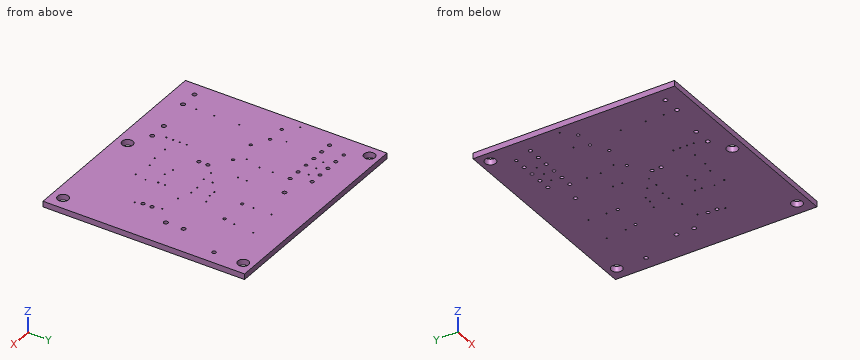
Autodesk Inventor part; units mm, degrees
ref_plane "YZ Plane" through (0, 0, 0) normal (1, 0, 0) x (0, 1, 0)
ref_plane "XZ Plane" through (0, 0, 0) normal (0, 1, 0) x (-1, 0, 0)
ref_plane "XY Plane" through (0, 0, 0) normal (0, 0, 1) x (1, 0, 0)
sketch "Sketch1" plane through (0, 0, 0) normal (0, 0, 1) x (1, 0, 0)
  line L0 (0, 0) -> (61.575, 0)
  line L1 (61.575, 0) -> (61.575, 56.82)
  line L2 (61.575, 56.82) -> (0, 56.82)
  line L3 (0, 56.82) -> (0, 0)
  circle A0 centre (10.16, 30.48) radius 0.405
  circle A1 centre (5.08, 30.48) radius 0.405
  circle A2 centre (22.23, 27.94) radius 0.405
  circle A3 centre (14.61, 27.94) radius 0.405
  circle A4 centre (44.45, 40.01) radius 0.405
  circle A5 centre (36.83, 40.01) radius 0.405
  circle A6 centre (27.3, 24.13) radius 0.51
  circle A7 centre (27.3, 21.59) radius 0.51
  circle A8 centre (49.53, 22.86) radius 0.51
  circle A9 centre (49.53, 20.32) radius 0.51
  circle A10 centre (27.3, 45.72) radius 0.55
  circle A11 centre (57.79, 45.72) radius 0.55
  circle A12 centre (4.57, 43.61) radius 0.5
  circle A13 centre (6.27, 48.69) radius 0.43
  circle A14 centre (7.98, 43.61) radius 0.5
  circle A15 centre (9.68, 48.69) radius 0.5
  circle A16 centre (11.38, 43.61) radius 0.5
  circle A17 centre (13.08, 48.69) radius 0.5
  circle A18 centre (14.78, 43.61) radius 0.43
  circle A19 centre (16.48, 48.69) radius 0.5
  circle A20 centre (18.19, 43.61) radius 0.5
  circle A21 centre (19.89, 48.69) radius 0.5
  circle A22 centre (21.59, 43.61) radius 0.5
  circle A23 centre (19.09, 6.35) radius 0.595
  circle A24 centre (24.09, 6.35) radius 0.595
  circle A25 centre (3.85, 5.08) radius 0.595
  circle A26 centre (8.85, 5.08) radius 0.595
  circle A27 centre (53.34, 34.25) radius 0.595
  circle A28 centre (53.34, 29.25) radius 0.595
  circle A29 centre (57.785, 3.175) radius 1.524
  circle A30 centre (3.175, 53.975) radius 1.524
  circle A31 centre (57.785, 53.975) radius 1.524
  circle A32 centre (29.845, 3.175) radius 1.524
  circle A33 centre (36.83, 27.305) radius 0.175
  circle A34 centre (39.37, 27.305) radius 0.175
  circle A35 centre (40.64, 32.385) radius 0.175
  circle A36 centre (20.32, 30.48) radius 0.175
  circle A37 centre (27.94, 33.02) radius 0.175
  circle A38 centre (27.94, 35.56) radius 0.175
  circle A39 centre (21.59, 34.925) radius 0.175
  circle A40 centre (21.59, 38.735) radius 0.175
  circle A41 centre (36.83, 43.18) radius 0.175
  circle A42 centre (45.085, 43.18) radius 0.175
  circle A43 centre (36.83, 48.26) radius 0.175
  circle A44 centre (45.72, 48.895) radius 0.175
  circle A45 centre (40.005, 20.32) radius 0.175
  circle A46 centre (40.005, 18.415) radius 0.175
  circle A47 centre (40.005, 12.065) radius 0.175
  circle A48 centre (31.75, 12.065) radius 0.175
  circle A49 centre (27.305, 12.065) radius 0.175
  circle A50 centre (8.89, 8.89) radius 0.175
  circle A51 centre (8.89, 13.97) radius 0.175
  circle A52 centre (8.89, 20.955) radius 0.175
  circle A53 centre (8.89, 34.29) radius 0.175
  circle A54 centre (1.905, 33.655) radius 0.175
  circle A55 centre (11.43, 46.355) radius 0.175
  circle A56 centre (14.605, 46.355) radius 0.175
  circle A57 centre (43.18, 26.035) radius 0.175
  circle A58 centre (50.165, 18.415) radius 0.175
  circle A59 centre (48.895, 25.4) radius 0.175
  circle A60 centre (33.655, 18.415) radius 0.175
  circle A61 centre (17.78, 46.355) radius 0.175
  circle A62 centre (33.02, 26.67) radius 0.175
  circle A63 centre (29.845, 26.67) radius 0.175
  circle A64 centre (33.02, 29.21) radius 0.175
  circle A65 centre (22.86, 9.525) radius 0.175
  circle A66 centre (22.86, 11.43) radius 0.175
  circle A67 centre (22.86, 13.335) radius 0.175
  circle A68 centre (22.86, 15.24) radius 0.175
  circle A69 centre (36.195, 31.75) radius 0.175
  circle A70 centre (34.925, 12.7) radius 0.175
  circle A71 centre (38.1, 31.75) radius 0.175
  circle A72 centre (40.64, 15.24) radius 0.175
  circle A73 centre (36.195, 17.78) radius 0.175
extrude "MPS_Drive_Amp_2.brd_Outline" add sketch "Sketch1" along normal blind 1.6
properties part number "MPS_Drive_Amp_2.brd_Outline"
Can you work these out from the model? Positions are in its coordinate system, mm. Give positions to 0.01 mm unless a question says otherwise; leave off trailing zeros. Use CSV: the item, a comma, the result in double quotes. Start each with the question number.
1. Imagine slicing it at A-A, the plane z = 1.2. Count the separate pieces of the cut face and the enclosed holes in it, plus the area to 3 significant figures.
2. If I drill on L1, parallel to X at y = 48.69, z = 0.9 (3 decimals); L2, parallel to X at y = 54, z = 0.9 (3 decimals); L3, parallel to Y at x = 11.43, z = 0.6, over which ranges is the centre line in solid material (lowest first)?
3. For P1, Ø1.5, axis at x = 24.09, y = 6.35, coming from the +Z side, with a flat end and sliding along its axis, tell me the tip position at first contact or that it passes through.
Response values:
1,separate pieces,"1"
1,enclosed holes,"74"
1,area,"3,440 mm^2"
2,L1,"0 to 5.84, 6.7 to 9.18, 10.18 to 12.58, 13.58 to 15.98, 16.98 to 19.39, 20.39 to 61.575"
2,L2,"0 to 1.651, 4.699 to 56.261, 59.309 to 61.575"
2,L3,"0 to 43.11, 44.11 to 46.18, 46.53 to 56.82"
3,P1,"z = 1.6"
